Autodesk Inventor part; units mm, degrees
ref_plane "YZ Plane" through (0, 0, 0) normal (1, 0, 0) x (0, 1, 0)
ref_plane "XZ Plane" through (0, 0, 0) normal (0, 1, 0) x (-1, 0, 0)
ref_plane "XY Plane" through (0, 0, 0) normal (0, 0, 1) x (1, 0, 0)
sketch "Sketch1" plane through (0, 0, 0) normal (0, 0, 1) x (1, 0, 0)
  circle A0 centre (-34, 4) radius 1.5
  circle A1 centre (-30, 13) radius 1.5
  circle A2 centre (-27, 4) radius 1.5
  line L0 (-30, 23) -> (-30, 40)
  line L1 (-39.076923, 9.384615) -> (-30, 23)
  line L2 (-40, 0) -> (-40, 8)
  line L3 (-40, 0) -> (-20, 0)
  line L4 (-20, 0) -> (-20, 40)
  line L5 (-20, 40) -> (-30, 40)
  circle A3 centre (-6, 4) radius 1.5
  circle A4 centre (-10, 13) radius 1.5
  circle A5 centre (-13, 4) radius 1.5
  line L6 (-10, 23) -> (-10, 40)
  line L7 (-20, 40) -> (-10, 40)
  line L8 (-20, 0) -> (-20, 40)
  line L9 (0, 0) -> (-20, 0)
  line L10 (0, 0) -> (0, 8)
  line L11 (-0.923077, 9.384615) -> (-10, 23)
  line L12 (-3, 8) -> (-37, 8)
  circle A6 centre (-29, 80.883435) radius 1.5
  circle A7 centre (-27, 90.883435) radius 1.5
  circle A8 centre (-35, 90.883435) radius 1.5
  line L13 (-40, 79.500979) -> (-40, 94.883435)
  arc A9 (-32.05, 74.283435) -> (-40, 79.500979) centre (-43.25, 65.883435) ccw
  line L14 (-28.021661, 68.912316) -> (-32.05, 74.283435)
  line L15 (-20, 68.912316) -> (-28.021661, 68.912316)
  line L16 (-20, 94.883435) -> (-20, 68.912316)
  line L17 (-40, 94.883435) -> (-20, 94.883435)
  circle A10 centre (-11, 80.883435) radius 1.5
  circle A11 centre (-13, 90.883435) radius 1.5
  circle A12 centre (-5, 90.883435) radius 1.5
  line L18 (0, 79.500979) -> (0, 94.883435)
  line L19 (0, 94.883435) -> (-20, 94.883435)
  line L20 (-20, 94.883435) -> (-20, 68.912316)
  line L21 (-20, 68.912316) -> (-11.978339, 68.912316)
  line L22 (-11.978339, 68.912316) -> (-7.95, 74.283435)
  arc A13 (0, 79.500979) -> (-7.95, 74.283435) centre (3.25, 65.883435) ccw
  line L23 (-10, 40) -> (-11.978339, 68.912316)
  line L24 (-28.021661, 68.912316) -> (-30, 40)
sketch "Sketch1 outline for Extrusion1" plane through (0, 0, 0) normal (0, 0, 1) x (1, 0, 0)
  line L0 (-37, 8) -> (-3, 8)
  line L1 (-30, 23) -> (-37, 8)
  line L2 (-3, 8) -> (-10, 23)
  line L3 (-30, 40) -> (-30, 23)
  line L4 (-10, 23) -> (-10, 40)
  line L5 (-28.021661, 68.912316) -> (-30, 40)
  line L6 (-10, 40) -> (-11.978339, 68.912316)
  line L7 (-32.05, 74.283435) -> (-28.021661, 68.912316)
  line L8 (-11.978339, 68.912316) -> (-7.95, 74.283435)
  arc A0 (-40, 79.500979) -> (-32.05, 74.283435) centre (-43.25, 65.883435) cw
  arc A1 (-7.95, 74.283435) -> (0, 79.500979) centre (3.25, 65.883435) cw
  line L9 (-40, 94.883435) -> (-40, 79.500979)
  line L10 (0, 79.500979) -> (0, 94.883435)
  line L11 (-20, 94.883435) -> (-40, 94.883435)
  line L12 (0, 94.883435) -> (-20, 94.883435)
  circle A2 centre (-30, 13) radius 1.5
  circle A3 centre (-10, 13) radius 1.5
  circle A4 centre (-29, 80.883435) radius 1.5
  circle A5 centre (-35, 90.883435) radius 1.5
  circle A6 centre (-27, 90.883435) radius 1.5
  circle A7 centre (-13, 90.883435) radius 1.5
  circle A8 centre (-11, 80.883435) radius 1.5
  circle A9 centre (-5, 90.883435) radius 1.5
extrude "Extrusion1" add sketch "Sketch1 outline for Extrusion1" along normal blind 2
chamfer "Chamfer1" distance 5 angle 45 2 edges at (-37, 8, 1) (-3, 8, 1)
sketch "Sketch2" plane through (0, 0, 2) normal (0, 0, 1) x (1, 0, 0)
  circle A0 centre (-27, 35.883435) radius 1.5
  circle A1 centre (-13, 35.883435) radius 1.5
  circle A2 centre (-13, 25.883435) radius 1.5
  circle A3 centre (-27, 25.883435) radius 1.5
  circle A4 centre (-20, 75.883435) radius 1.5
  circle A5 centre (-20, 25.883435) radius 1.5
  circle A6 centre (-20, 15.883435) radius 1.5
  circle A7 centre (-20, 35.883435) radius 1.5
  circle A8 centre (-20, 85.883435) radius 1.5
  line L0 (-5, 8) -> (-2.773501, 12.160251)
  line L1 (-5, 8) -> (-35, 8)
  line L2 (-37.226499, 12.160251) -> (-35, 8)
  line L3 (-37.226499, 12.160251) -> (-30, 23)
  line L4 (-30, 23) -> (-30, 40)
  line L5 (-30, 40) -> (-26, 40)
  arc A9 (-26, 40) -> (-23, 43) centre (-26, 43) ccw
  line L6 (-23, 43) -> (-23, 65.912316)
  arc A10 (-23, 65.912316) -> (-26, 68.912316) centre (-26, 65.912316) ccw
  line L7 (-26, 68.912316) -> (-28.021661, 68.912316)
  line L8 (-28.021661, 68.912316) -> (-32.05, 74.283435)
  arc A11 (-32.05, 74.283435) -> (-40, 79.500979) centre (-43.25, 65.883435) ccw
  line L9 (-40, 79.500979) -> (-40, 94.883435)
  line L10 (-40, 94.883435) -> (0, 94.883435)
  line L11 (0, 94.883435) -> (0, 79.500979)
  arc A12 (0, 79.500979) -> (-7.95, 74.283435) centre (3.25, 65.883435) ccw
  line L12 (-7.95, 74.283435) -> (-11.978339, 68.912316)
  line L13 (-11.978339, 68.912316) -> (-14, 68.912316)
  arc A13 (-14, 68.912316) -> (-17, 65.912316) centre (-14, 65.912316) ccw
  line L14 (-17, 65.912316) -> (-17, 43)
  arc A14 (-17, 43) -> (-14, 40) centre (-14, 43) ccw
  line L15 (-14, 40) -> (-10, 40)
  line L16 (-10, 40) -> (-10, 23)
  line L17 (-10, 23) -> (-2.773501, 12.160251)
  circle A15 centre (-30, 13) radius 1.5
  circle A16 centre (-27, 90.883435) radius 1.5
  circle A17 centre (-29, 80.883435) radius 1.5
  circle A18 centre (-35, 90.883435) radius 1.5
  circle A19 centre (-11, 80.883435) radius 1.5
  circle A20 centre (-13, 90.883435) radius 1.5
  circle A21 centre (-5, 90.883435) radius 1.5
  circle A22 centre (-10, 13) radius 1.5
  point P0 (0, 0)
extrude "Extrusion2" cut sketch "Sketch2" against normal blind 10 contours A0 | A1 | A2 | A3 | A4 | A5 | A6 | A7 | A8
sketch "Sketch3" plane through (0, 0, 2) normal (0, 0, 1) x (1, 0, 0)
  circle A0 centre (-13, 35.883435) radius 1.5
  circle A1 centre (-20, 35.883435) radius 1.5
  circle A2 centre (-27, 35.883435) radius 1.5
  circle A3 centre (-13, 25.883435) radius 1.5
  circle A4 centre (-20, 75.883435) radius 1.5
  circle A5 centre (-20, 25.883435) radius 1.5
  circle A6 centre (-27, 25.883435) radius 1.5
  circle A7 centre (-20, 15.883435) radius 1.5
  circle A8 centre (-20, 85.883435) radius 1.5
  line L0 (-5.114427, 12.530916) -> (-8, 8)
  line L1 (-5.114427, 12.530916) -> (-10, 23)
  line L2 (-10, 23) -> (-10, 40)
  line L3 (-10, 40) -> (-11.978339, 68.912316)
  line L4 (-11.978339, 68.912316) -> (-7.95, 74.283435)
  arc A9 (0, 79.500979) -> (-7.95, 74.283435) centre (3.25, 65.883435) ccw
  line L5 (0, 79.500979) -> (0, 94.883435)
  line L6 (0, 94.883435) -> (-40, 94.883435)
  line L7 (-40, 94.883435) -> (-40, 79.500979)
  arc A10 (-32.05, 74.283435) -> (-40, 79.500979) centre (-43.25, 65.883435) ccw
  line L8 (-32.05, 74.283435) -> (-28.021661, 68.912316)
  line L9 (-28.021661, 68.912316) -> (-30, 40)
  line L10 (-30, 40) -> (-30, 23)
  line L11 (-30, 23) -> (-34.885573, 12.530916)
  line L12 (-32, 8) -> (-34.885573, 12.530916)
  line L13 (-32, 8) -> (-8, 8)
  circle A11 centre (-13, 90.883435) radius 1.5
  circle A12 centre (-11, 80.883435) radius 1.5
  circle A13 centre (-5, 90.883435) radius 1.5
  circle A14 centre (-29, 80.883435) radius 1.5
  circle A15 centre (-27, 90.883435) radius 1.5
  circle A16 centre (-35, 90.883435) radius 1.5
  circle A17 centre (-30, 13) radius 1.5
  circle A18 centre (-10, 13) radius 1.5
  circle A19 centre (-20, 75.883435) radius 1.5
  line L14 (-20, 75.883435) -> (-20, 55.883435)
  line L15 (-20, 55.883435) -> (-20, 45.883435)
  circle A20 centre (-20, 55.883435) radius 1.5
  circle A21 centre (-20, 45.883435) radius 1.5
  point P0 (0, 0)
  dimension "d7" = 20
  dimension "d8" = 10
  dimension "d9" = 3
  dimension "d10" = 3
extrude "Extrusion3" cut sketch "Sketch3" against normal blind 10 contours A20 L15 L14 | L14 L15 A20 | A21
properties part number "body_bone_3"
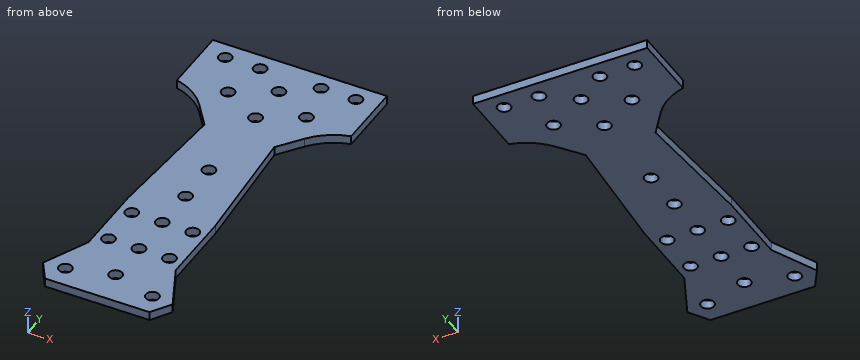
The model under review builds one solid part; all positions refer to its coordinate system, in mm. Give positions to 0.01 mm unless a question says otherwise; leave off trailing zeros. Loops run counter-clockwise (first coordinate to the right, second up) from the corner with the lowest first, then second, coordinate; pieces in that order, holes last. Notation, with made-up numbers: (-36, 52.25) -> (1, 52.25) arc R26 ccw to (1, 81.25) -> close; hole circle Ø11 at (30, -30.5). An arc over 180 degrees is marked (long way). Answer as a JSON object with one key per item and string values. Group by question number.
Q1. Wall thickness on line 1 along Y through (x, z) = (-13, 1.2); line 2 along X through (y, z) = (91, 1.15); line 3 along X through (y, z) = (37, 0.25): over which ranges is each line inside the solid? List them lowest first.
Q2. Take a section at A-A (x = -20). State how many separate pieces and enclosed holes the cut face has, plus the area to 3 significant figures.
Q3. Take a section at C-C (y = 21). Write out the cut boundary in (x, z), plus the area to 3 significant figures.
Answer below:
{
 "1": {"line 1": "y = 8 to 24.38, 27.38 to 34.38, 37.38 to 89.38, 92.38 to 94.88", "line 2": "x = -40 to -36.5, -33.5 to -28.5, -25.5 to -14.5, -11.5 to -6.5, -3.5 to 0", "line 3": "x = -30 to -28, -26 to -21, -19 to -14, -12 to -10"},
 "2": {"separate pieces": "8", "enclosed holes": "0", "area": "132 mm2"},
 "3": {"outline": "(-30.93, 0) -> (-9.07, 0) -> (-9.07, 2) -> (-30.93, 2) -> close", "area": "43.7 mm2"}
}
